from build123d import *

# Parameters (mm, degrees)
F2_DEPTH = 43.434
F3_DEPTH = 37.084
F4_DEPTH = 16.002
F5_DEPTH = 42.672
F6_DEPTH = 44.45
F7_DEPTH = 25.4
F8_DEPTH = 25.4


with BuildPart() as f2:
    # F1 (on Right) → F2 (new body)
    with BuildSketch(Plane.YZ):
        Polygon((-16.6454371065, 0), (0, -56.3706830144), (0, 0), (0, 55.5314160883), align=None)
    extrude(amount=-F2_DEPTH)

    # F3 (add): a face of the model
    f3_faces = [f2.faces().sort_by_distance(p)[0] for p in [
        (0, -5.5484790355, -0.279755642),
    ]]
    extrude(f3_faces, amount=F3_DEPTH)

    # F0 (on Front) → F4 (join)
    with BuildSketch(Plane.XZ):
        Polygon((0, 56.3706830144), (-34.2700183392, 0), (0, -56.3706830144), (34.2700183392, 0), align=None)
    extrude(amount=-F4_DEPTH)

    # F5 (add): a face of the model
    f5_faces = [f2.faces().sort_by_distance(p)[0] for p in [
        (-17.1350091696, 8.001, -28.1853415072),
    ]]
    extrude(f5_faces, amount=F5_DEPTH)

    # F6 (add): a face of the model
    f6_faces = [f2.faces().sort_by_distance(p)[0] for p in [
        (17.1350091696, 8.001, -28.1853415072),
    ]]
    extrude(f6_faces, amount=F6_DEPTH)

    # F7 (cut): a face of the model
    f7_faces = [f2.faces().sort_by_distance(p)[0] for p in [
        (-28.7931585995, 0, 33.1465043739),
    ]]
    extrude(f7_faces, amount=-F7_DEPTH, mode=Mode.SUBTRACT)

    # F8 (cut): a face of the model
    f8_faces = [f2.faces().sort_by_distance(p)[0] for p in [
        (24.8505885604, 0, 35.6188502379),
    ]]
    extrude(f8_faces, amount=-F8_DEPTH, mode=Mode.SUBTRACT)


solid = f2.part
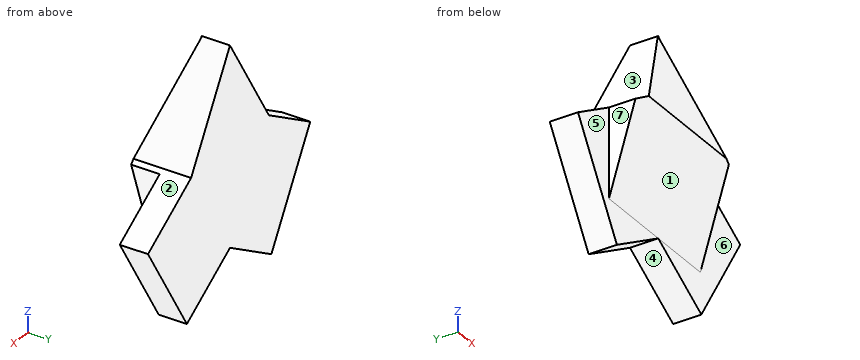
The listing builds one solid part. Answer for the finished solid, in the listing's coordinates (mm). Face numbers are marked on the shaded views. A direction names the side the tool comes from. Coordinates: 2 decimals unless noted, no trailing zeros. Write each loop counter-clockwise with the first axis right and the second up, starting at its lowest first coordinate (ties: lowest second). Pieces come first, ordered by that corner, then holes. Notation, with made-up numbers: (78.5, 25) -> (102.5, 25) arc R9 ccw to (102.5, 36) -> close; hole circle Ø6 at (19, -13). An arc over 180 degrees is marked (long way). One line per question, with ' | ' between items.
1. Which of the six approach directions +Z, -Z, +X, -X, +Y, -Y give full straight-line access (tool end or side, diameter ignored) to the marked faces 5, 6 and 7?
Verdict:
face 5: -Z, -X, -Y | face 6: -Z, +X, -Y | face 7: +Z, -Z, -X, -Y
2. Given pin 1 Ø10 at (x, y) = (37.5, 2) entering from +Z; pin 2 Ø2 at (x, y) = (-19, -7.5) entering from +Z; pin 3 Ø12 at (x, y) = (4, 3.5) entering from -Z, each flat-ended and moving along its own axis, determine where each tip first touches the part or whether it passes through.
Verdict:
pin 1: stops at z = 2.91 | pin 2: stops at z = 26.76 | pin 3: stops at z = -62.45
3. Section C-C (z = -40.5) is taken. Determine the outline of the cut face in (x, y).
Verdict:
outline: (-59.59, 0) -> (-43.43, 0) -> (-43.43, -4.69) -> (37.08, -4.69) -> (37.08, 0) -> (61.67, 0) -> (61.67, 16) -> (-59.59, 16) -> close
4. Section D-D (x = -22.5) is taken. Determine the outline of the cut face in (y, z).
Verdict:
outline: (-16.65, 0) -> (0, -56.37) -> (0, -70.05) -> (16, -70.05) -> (16, 19.36) -> (-10.84, 19.36) -> close
5. Section B-B (y = 11.5) is taken. Determine the outline of the cut face in (x, z), and give its area (3 significant figures).
Verdict:
outline: (-70.73, -22.17) -> (-36.46, -78.54) -> (0, -56.37) -> (37.98, -79.46) -> (72.25, -23.09) -> (34.27, 0) -> (0, 56.37) -> (-34.27, 0) -> close | area: 9,610 mm^2
6. Straight lines are drawn through the part: line 1 (Y direction, x = 55, z = -16); line 2 (X direction, y = 1.5, z = -69); line 3 (Y direction, x = 27, z = -5.5). For each, find the intervals that lie inside material, in ascending order.
Verdict:
line 1: y = 0 to 16 | line 2: x = -42.26 to -20.77, 20.77 to 44.34 | line 3: y = -15.02 to 16
7. For a pull along X with two mould halves and no side action, classify the marked faces 1, 2, 3 and 4 as released by +X, released by -X, zero draft, split by the parting line, or undercut.
Verdict:
face 1: zero draft | face 2: released by +X | face 3: released by -X | face 4: undercut
8. Section A-A (z = -61.5) is taken. Determine the outline of the cut face in (x, y).
Verdict:
outline: (-46.82, 0) -> (-8.44, 0) -> (-8.44, 16) -> (-46.82, 16) -> close; (8.44, 0) -> (48.9, 0) -> (48.9, 16) -> (8.44, 16) -> close
